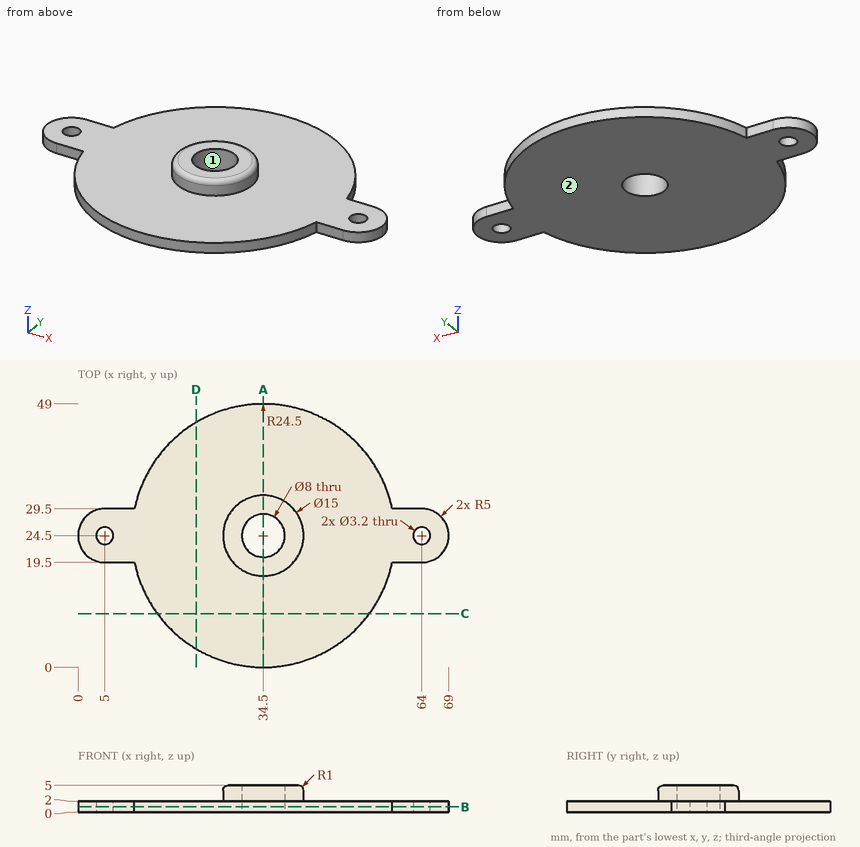
Geometry: see drawing. Coordinates: mm, zero at the bounding-box minimum. Coordinates: 2 decimals unless noted, no trailing zeros. Order: outer loops, then holes, each group sorted by start corner. A loop starts at its lowest first (then second) coordinate and runs counter-clockwise, first axis right, second up. Notation, with made-up numbers: (-9.5, 1.5) - (36.5, 1.5) arc R23 cw to (36.5, 17.5) - close; hole circle Ø7 at (-38.5, -28.75). An arc over 180 degrees is marked (long way). Use one line per item in the form item = value.
1) Section A-A (x = 34.5). Return loops of the section in (y, z), then the cut area to 3 significant figures.
Solutions:
outline = (0, 0) - (20.5, 0) - (20.5, 5) - (18, 5) arc R1 ccw to (17, 4) - (17, 2) - (0, 2) - close; (28.5, 0) - (49, 0) - (49, 2) - (32, 2) - (32, 4) arc R1 ccw to (31, 5) - (28.5, 5) - close
area = 103 mm^2
2) Pin query (flat end, axial travel): pin 1 (13 mm diameter, centred on x = 34.5, y = 24.5, fed in from +Z); pin 2 (1 mm diameter, centred on x = 32, z = 4, fed in from +Y); pin 3 (1 mm diameter, centred on x = 61, z = 1, fed in from +Y); pin 4 (3 mm diameter, centred on x = 44.5, z = 4, fed in from -Y). Return the tip coordinate at first contact, or that it passes through.
Solutions:
pin_1 = 5
pin_2 = 31.73
pin_3 = 29.5
pin_4 = through
3) Mould query, pull axis Y, two halves, no side actions, for the marked faces 1 and 2. Classes: +Y half, -Y half, draft (parallel to the pull), parting line (faces both ways), or undercut.
Solutions:
face_1 = undercut
face_2 = draft
4) Section B-B (z = 1). Return loops of the section in (x, y).
Solutions:
outline = (5, 19.5) - (10.52, 19.5) arc R24.5 ccw to (58.48, 19.5) - (64, 19.5) arc R5 ccw to (64, 29.5) - (58.48, 29.5) arc R24.5 ccw to (10.52, 29.5) - (5, 29.5) arc R5 ccw to start; hole circle Ø3.2 at (5, 24.5); hole circle Ø8 at (34.5, 24.5); hole circle Ø3.2 at (64, 24.5)
5) Ray query, L1, parallel to Y at x = 59, z = 0.4; L2, parallel to Y at x = 5, z = 1.5; L3, parallel to Z at x = 48, y = 20.5. Return the intervals inside material, ascending.
Solutions:
L1 = 19.5 to 29.5
L2 = 19.5 to 22.9, 26.1 to 29.5
L3 = 0 to 2
6) Section D-D (x = 22). Return loops of the section in (y, z).
Solutions:
outline = (3.43, 0) - (45.57, 0) - (45.57, 2) - (3.43, 2) - close
7) Section C-C (y = 10). Return loops of the section in (x, z), then the cut area to 3 significant figures.
Solutions:
outline = (14.75, 0) - (54.25, 0) - (54.25, 2) - (14.75, 2) - close
area = 79.0 mm^2
